Build history of the part. All positions in model axes, mm. A direction names the side the tool comes from. Coordinates: 2 decimals unless noted, no trailing zeros. Loops run counter-clockwise (first coordinate to the right, second up) from the corner with the lowest first, then second, coordinate; pieces in that order, holes last. Notation, with made-up numbers: (42, 3.25) - (96, 3.25) arc R32 cw to (96, 36.25) - close; hole circle Ø3 at (1, 7). An arc over 180 degrees is marked (long way). One line per item, written item: value.
Autodesk Inventor part; units mm, degrees
ref_plane "YZ Plane" through (0, 0, 0) normal (1, 0, 0) x (0, 1, 0)
ref_plane "XZ Plane" through (0, 0, 0) normal (0, 1, 0) x (-1, 0, 0)
ref_plane "XY Plane" through (0, 0, 0) normal (0, 0, 1) x (1, 0, 0)
sketch "Szkic1" plane through (0, 0, 0) normal (0, 0, 1) x (1, 0, 0)
  line L0 (0, 0) -> (77, 0)
  line L1 (77, 0) -> (77, 50)
  line L2 (77, 50) -> (0, 50)
  line L3 (0, 50) -> (0, 0)
  dimension "d0" = 77
  dimension "d1" = 50
extrude "Wyciągnięcie proste1" add sketch "Szkic1" along normal blind 10
sketch "Szkic2" plane through (0, 0, 0) normal (0, -1, 0) x (1, 0, 0)
  line L0 (77, 0) -> (0, 0)
  line L1 (0, 0) -> (77, 0)
  line L2 (77, 0) -> (0, 0)
  line L3 (0, 0) -> (0, -10)
  line L4 (0, -10) -> (73.2222, -10)
  line L5 (77, 0) -> (0, 0)
  line L6 (73.2222, -10) -> (77, 0)
  dimension "d6" = 10
extrude "Wyciągnięcie proste2" add sketch "Szkic2" against normal blind 50
sketch "Szkic3" plane through (0, 50, 10) normal (0, 1, 0) x (1, 0, 0)
  line L0 (0, 20) -> (0, 0)
  line L1 (0, 20) -> (0, 38)
  line L2 (77, 10) -> (73.2222, 20)
  line L3 (73.2222, 20) -> (66.4222, 38)
  line L4 (66.4222, 38) -> (0, 38)
  point P0 (0, 10)
  dimension "d9" = 18
sketch "Szkic4" plane through (0, 50, 10) normal (0, 1, 0) x (1, 0, 0)
  line L0 (0, 20) -> (0, 0)
  line L1 (0, 20) -> (0, 38)
  line L2 (73.2222, 20) -> (0, 20)
  line L3 (0, 20) -> (73.2222, 20)
  line L4 (73.2222, 20) -> (65.2222, 38)
  line L5 (65.2222, 38) -> (0, 38)
  point P0 (0, 10)
  dimension "d10" = 18
extrude "Wyciągnięcie proste3" add sketch "Szkic4" against normal blind 15
sketch "Szkic5" plane through (0, 50, 10) normal (0, 1, 0) x (1, 0, 0)
  line L0 (0, 38) -> (65.2222, 38)
  line L1 (0, 38) -> (0, 55)
  line L2 (0, 38) -> (65.2222, 38)
  line L3 (65.2222, 38) -> (73.2222, 20)
  line L4 (57.6666, 55) -> (65.2222, 38)
  line L5 (0, 55) -> (14, 55)
  line L6 (14, 55) -> (14, 45)
  line L7 (14, 45) -> (49, 45)
  line L8 (49, 45) -> (49, 55)
  line L9 (49, 55) -> (57.6666, 55)
  point P0 (0, 10)
  dimension "d13" = 17
  dimension "d14" = 14
  dimension "d15" = 10
  dimension "d16" = 35
extrude "Wyciągnięcie proste4" add sketch "Szkic5" against normal blind 30
Item 1: Pull direction Z, two halves, no side cores. Call faces 1 (the face through (36, 17, -10)), 2 (the face through (32.2, 20, -34.7)), 3 (the face through (38, 25, 10)): released by +Z, released by -Z, zero draft, split by the parting line, or undercut.
Check result:
face 1: undercut
face 2: zero draft
face 3: released by +Z
Item 2: Cut at A-A, the plane x = 52.5. Write the cut outline in (y, z).
Check result:
outline: (0, -10) - (35, -10) - (35, -28) - (20, -28) - (20, -45) - (50, -45) - (50, 10) - (0, 10) - close
Item 3: Tool access for faces 4 (the face through (32, 28, -28)), 5 (the face through (38, 0, 0)), 6 (the face through (31, 35, -35)): list every direction of +Z, -Z, +X, -X, +Y, -Y with a clear straight run to the whole face (end or side of a thin tool).
Check result:
face 4: +X, -X, -Y
face 5: +Z, -Z, +X, -X, -Y
face 6: -Z, +Y, -Y
Item 4: Drop flat-ended pins along their axis: P1, Ø8, axis at x = 36.5, y = 7, coming from the -Z side; P2, Ø8, axis at x = 62.5, y = 41.5, coming from the -Z side; P3, Ø5, axis at y = 33, z = -40, coming from the +X side; P4, Ø1, axis at y = 39.5, z = -29.5, coming from the -X side. Give the stop position or say it passes through.
Check result:
P1: stops at z = -10
P2: stops at z = -43.12
P3: stops at x = 61
P4: stops at x = 0
Item 5: Cut at C-C, the plane x = 34. Write the cut outline in (y, z), then the cut area to 3 significant figures.
Check result:
outline: (0, -10) - (35, -10) - (35, -28) - (20, -28) - (20, -35) - (50, -35) - (50, 10) - (0, 10) - close
area: 1,480 mm^2
Item 6: Cut at B-B, the plane y = 16. Write the cut outline in (x, z), then the cut area to 3 significant figures.
Check result:
outline: (0, -10) - (73.22, -10) - (77, 0) - (77, 10) - (0, 10) - close
area: 1,520 mm^2
Item 7: Cut at D-D, the plane z = -27. Write the cut outline in (x, y), then the cut area to 3 significant figures.
Check result:
outline: (0, 35) - (65.67, 35) - (65.67, 50) - (0, 50) - close
area: 985 mm^2
Item 8: Probe probe 1 along Z at (x, y) = (17, 29.5); probe 2 along Z at (x, y) = (53.5, 34); probe 3 along Z at (x, y) = (6, 7.5). List the from-to ranges inside material, lowest first. Write a range as from..to.
Check result:
probe 1: z = -35..-28, -10..10
probe 2: z = -45..-28, -10..10
probe 3: z = -10..10
